The model under review builds one solid part; all positions refer to its coordinate system, in mm. Round coordinates to 2 decimals unless told otherwise and drop trailing zeros. Order: outer loops, then holes, each group sorted by start corner. A loop starts at its lowest first (then second) coordinate and runs counter-clockwise, first axis right, second up. Notation, with made-up numbers: (29, 55) - (88, 55) arc R11 cw to (88, 70) - close; hole circle Ø4 at (-24.75, 69.25). An arc over 180 degrees is marked (long way). One line per question, with ' | ' between items. Start each with the question number.
Item 1: For L1, parallel to X at y = 0, z = 87; L2, parallel to X at y = 23, z = 94.5, list the stretches that pass through material, from the lowest coordinate up. Write a range as [from, to].
Item 2: Draft analysis for pull direction Y (two halves, no side actions). For faces 1 (the face through (-11, 5, 0)), 2 (the face through (8.071, -15.518, 18.744)), 3 (the face through (27.712, -11.49, 77.159)), 4 (the face through (24.94, -10.34, 77.16)), state which applies: +Y half, -Y half, draft (parallel to the pull), parting line (faces both ways), or undercut.
Item 3: Add section B-B on z = 22. State the section outline as (x, y) points.
Item 4: Insertion check: pin 1 Ø4 at (y, z) = (-20, 18) entering from +X; pin 2 Ø2 at (y, z) = (5, 80) entering from +X; pin 3 Ø4 at (y, z) = (19, 35.5) entering from +X. Each pin has a flat end and moves straight along its axis. Give the tip position at first contact, or say it passes through.
Item 5: Add section A-A on z = 61.5. State the section outline as (x, y) points, and give its area (3 significant figures).
from build123d import *

# Parameters (mm, degrees)
F2_R = 25
F3_T = -3


with BuildPart() as f1:
    # F0 (on Front) → F1 (revolve)
    with BuildSketch(Plane.XZ):
        Polygon((0, 100), (0, 0), (15, 0), (30, 50), (30, 100), align=None)
    revolve(axis=Axis((0, 0, 50), (0, 0, 1)))

    # F2
    f2_edges = [f1.edges().sort_by_distance(p)[0] for p in [
        (-30, 0, 50),
    ]]
    fillet(f2_edges, radius=F2_R)

    # F3
    f3_openings = [f1.faces().sort_by_distance(p)[0] for p in [
        (0, 0, 100),
        (0, 0, 0),
    ]]
    offset(amount=F3_T, openings=f3_openings)


solid = f1.part
Determined:
1) L1: [-30, -27], [27, 30] | L2: [-19.26, -14.14], [14.14, 19.26]
2) face 1: draft | face 2: undercut | face 3: parting line | face 4: undercut
3) outline: circle Ø43.2 at (0, 0); hole circle Ø36.94 at (0, 0)
4) pin 1: x = 9.81 | pin 2: x = 29.73 | pin 3: x = 19.38
5) outline: circle Ø60 at (0, 0); hole circle Ø54 at (0, 0) | area: 537 mm2
